Autodesk Inventor part; units mm, degrees
ref_plane "YZ Plane" through (0, 0, 0) normal (1, 0, 0) x (0, 1, 0)
ref_plane "XZ Plane" through (0, 0, 0) normal (0, 1, 0) x (-1, 0, 0)
ref_plane "XY Plane" through (0, 0, 0) normal (0, 0, 1) x (1, 0, 0)
sketch "スケッチ1" plane through (0, 0, 0) normal (0, 1, 0) x (-1, 0, 0)
  line L0 (-5.2, 8) -> (-5.8, 8)
  line L1 (-6, 7.8) -> (-6, 0.2)
  line L2 (-5.8, 0) -> (-5.2, 0)
  line L3 (-5, 0.2) -> (-5, 7.8)
  line L4 (-5, 8) -> (-6, 0) construction
  line L5 (-6, 8) -> (-5, 0) construction
  line L6 (0, -1.6) -> (0, 9.6)
  line L7 (-5.8, 8) -> (-6, 7.8)
  line L8 (-6, 0.2) -> (-5.8, 0)
  line L9 (-5.2, 0) -> (-5, 0.2)
  line L10 (-5, 7.8) -> (-5.2, 8)
  point P0 (0, 0)
  point P1 (-5.5, 4)
  dimension "d0" = 10
  dimension "d1" = 12
  dimension "d2" = 8
  dimension "d3" = 0.2
  dimension "d4" = 0.2
  dimension "d5" = 0.2
  dimension "d6" = 0.2
  dimension "d7" = 0.2
  dimension "d8" = 0.2
  dimension "d9" = 0.2
  dimension "d10" = 0.2
revolve "回転1" add sketch "スケッチ1" angle 360 about axis through (0, 0, -10) along (0, 0, 1)
equation "\"d4\" = d3"
equation "\"d5\" = d3"
equation "\"d6\" = d5"
equation "\"d7\" = d3"
equation "\"d8\" = d7"
equation "\"d9\" = d3"
equation "\"d10\" = d9"
properties part number "WSSS-12-10-8" material "ステンレス鋼 AISI 304"
Work out the finished part from the listing and answer in its coordinate system (mm). Round coordinates to 2 decimals unless told otherwise and drop trailing zeros. Loops run counter-clockwise (first coordinate to the right, second up) from the corner with the lowest first, then second, coordinate; pieces in that order, holes last. Notation, with made-up numbers: (68.5, 41) -> (114.5, 41) arc R19 cw to (114.5, 77) -> close; hole circle Ø1 at (4.25, -39). An arc over 180 degrees is marked (long way). Write each question's results on one line, items separated by ' | '. Start each with the question number.
1. Given pin 1 Ø3 at (x, y) = (0, -2.5) entering from -Z; pin 2 Ø4 at (y, z) = (3, 7) entering from -X; pin 3 Ø1.5 at (x, z) = (2.5, 1.5) entering from +Y, each flat-ended and moving along its own axis, determine where each tip first touches the part or whether it passes through.
2. Section A-A (y = 0) is taken. Determine the outline of the cut face in (x, z), plus the area to 3 significant figures.
3. Find the intervals of material crossed by probe 1 along Y at (x, z) = (0, 5); probe 2 along Y at (x, z) = (3.75, 7); probe 3 along X at (y, z) = (-3, 2.25), in increasing order. Write a range as from..to.
4. For a pull along Y with two mould halves and no side action, classify faces 1 (the face through (-6, 0, 4)), 2 (the face through (-2, 5, 0)), 3 (the face through (-1.08, -4.88, 4.05)) as +Y half, -Y half, draft (parallel to the pull), parting line (faces both ways), or undercut.
5. Section C-C (z = 0.5) is taken. Determine the outline of the cut face in (x, y), plus the area to 3 significant figures.
Evaluation:
1) pin 1: passes through | pin 2: stops at x = -5.92 | pin 3: stops at y = 5.74
2) outline: (-6, 0.2) -> (-5.8, 0) -> (-5.2, 0) -> (-5, 0.2) -> (-5, 7.8) -> (-5.2, 8) -> (-5.8, 8) -> (-6, 7.8) -> close; (5, 0.2) -> (5.2, 0) -> (5.8, 0) -> (6, 0.2) -> (6, 7.8) -> (5.8, 8) -> (5.2, 8) -> (5, 7.8) -> close | area: 15.8 mm2
3) probe 1: y = -6..-5, 5..6 | probe 2: y = -4.68..-3.31, 3.31..4.68 | probe 3: x = -5.2..-4, 4..5.2
4) face 1: parting line | face 2: draft | face 3: undercut
5) outline: circle Ø12 at (0, 0); hole circle Ø10 at (0, 0) | area: 34.6 mm2
